Could you check a few things on this model? Use its own coordinates, in mm. Face numbers are marked on the shaded views. A direction names the side the tool comes from. Give positions to 0.01 mm unless a question says otherwise; leave off trailing zeros. Loops run counter-clockwise (first coordinate to the right, second up) from the corner with the lowest first, then second, coordinate; pieces in that order, holes last. Notation, with made-up numbers: M -8,8.5 L 14,8.5 A21 cw 14,44.5 Z; hole C 31.5,7.5 d7. An arc over 180 degrees is marked long. Answer in a Markdown table with one row per item. Add a question column.
1. If we section it at B-B on x = -8: List the corners of the cut face in (y, z) for me.
2. I'm going to push flat-ended pins straight in: pin 1 Ø1.8 at (x, z) = (-30, -45) entering from +Y; pin 2 Ø4.5 at (y, z) = (8, -41) entering from -X; pin 3 Ø7 at (x, z) = (-29, -39.5) entering from -Y; pin 4 Ø0.7 at (x, z) = (30, -45) entering from +Y. Where does each tip first touch, or does it pass through?
3. I need wall thicknesses on line 1 along X through (y, z) = (29.75, -45); line 2 along Z through (x, y) = (26, 15); line 3 along X through (y, z) = (24.5, 24.5). Which ranges of each line are inside material? Lowest first, please. Write a range as from..to.
4. Thinking about a two-plate mould opening in X: for the marked faces 5, 6, 7 and 8, which applies, released by +X, released by -X, zero draft, split by the parting line, or undercut?
5. Which directions (+Z, -Z, +X, -X, +Y, -Y) give clear straight access to the entire face, cutting with the end or side of a thin tool? Please do the marked faces 1, 2, 3 and 4.
6. If we section it at D-D on z = 19: List the corners of the cut face in (x, y) for me.
7. If we section it at A-A on y = 22: List the corners of the cut face in (x, z) for me, then the cut area to 3 significant figures.
8. If we section it at C-C on z = -42: List the corners of the cut face in (x, y) for me, then the cut area to 3 significant figures.
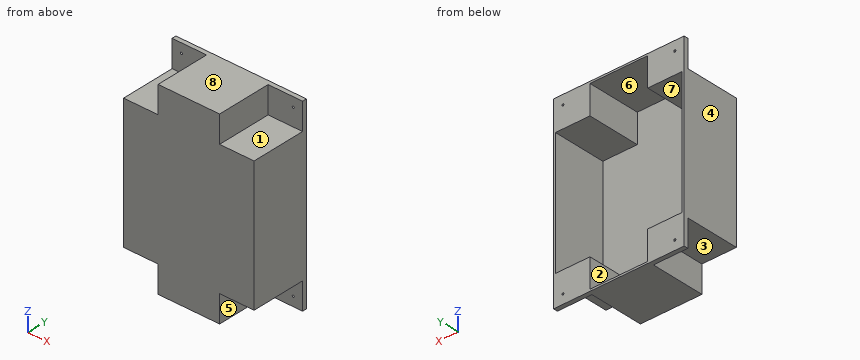
```python
from build123d import *

# Parameters (mm, degrees)
CROQUIS1_W              = 70
CROQUIS1_H              = 100
SALIENTE_EXTRUIR1_DEPTH = 3
CROQUIS2_W              = 70
CROQUIS2_H              = 100
SALIENTE_EXTRUIR2_DEPTH = 28.5
CROQUIS3_R              = 0.56
CORTAR_EXTRUIR1_DEPTH   = 69.682239334
CROQUIS4_W              = 18.5
CROQUIS4_H              = 14.45
CORTAR_EXTRUIR2_DEPTH   = 29.2


with BuildPart() as part:
    # Croquis1 → Saliente-Extruir1 (new body)
    with BuildSketch(Plane(origin=(0, 0, 0), x_dir=(1, 0, 0), z_dir=(0, 1, 0))):
        Rectangle(CROQUIS1_W, CROQUIS1_H)
    extrude(amount=SALIENTE_EXTRUIR1_DEPTH)

    # Croquis2 → Saliente-Extruir2 (add)
    with BuildSketch(Plane(origin=(0, 3, 0), x_dir=(1, 0, 0), z_dir=(0, 1, 0))):
        Rectangle(CROQUIS2_W, CROQUIS2_H)
        Polygon((-34, 33.55), (-15.5, 33.55), (-15.5, 49), (15.5, 49), (15.5, 33.55), (34, 33.55), (34, -33.55), (15.5, -33.55), (15.5, -49), (-15.5, -49), (-15.5, -33.55), (-34, -33.55), align=None, mode=Mode.SUBTRACT)
    extrude(amount=SALIENTE_EXTRUIR2_DEPTH)

    # Croquis3 → Cortar-Extruir1 (cut, through all)
    with BuildSketch(Plane.XZ):
        with Locations(Location((-30, -45, 0), (0, 0, 270))):
            Circle(CROQUIS3_R)
        with Locations(Location((-30, 45, 0), (0, 0, 90))):
            Circle(CROQUIS3_R)
        with Locations(Location((30, -45, 0), (0, 0, 90))):
            Circle(CROQUIS3_R)
        with Locations(Location((30, 45, 0), (0, 0, 270))):
            Circle(CROQUIS3_R)
    extrude(amount=-CORTAR_EXTRUIR1_DEPTH, mode=Mode.SUBTRACT)

    # Croquis4 → Cortar-Extruir2 (cut)
    with BuildSketch(Plane.XZ):
        with Locations((-25.75, 42.775)):
            Rectangle(CROQUIS4_W, CROQUIS4_H)
        with Locations((25.75, 42.775)):
            Rectangle(CROQUIS4_W, CROQUIS4_H)
        with Locations((25.75, -42.775)):
            Rectangle(CROQUIS4_W, CROQUIS4_H)
        with Locations((-25.75, -42.775)):
            Rectangle(CROQUIS4_W, CROQUIS4_H)
    extrude(amount=-CORTAR_EXTRUIR2_DEPTH, mode=Mode.SUBTRACT)


solid = part.part
```
Results:
| question | item | result |
|---|---|---|
| 1 | outline | M 0,-50 L 31.5,-50 L 31.5,-49 L 3,-49 L 3,49 L 31.5,49 L 31.5,50 L 0,50 Z |
| 2 | pin 1 | y = 31.5 |
| 2 | pin 2 | x = -16.5 |
| 2 | pin 3 | y = 29.2 |
| 2 | pin 4 | through |
| 3 | line 1 | -35..-30.56, -29.44..-15.5, 15.5..29.44, 30.56..35 |
| 3 | line 2 | -35.55..-33.55, 33.55..35.55 |
| 3 | line 3 | -35..-34, 34..35 |
| 4 | face 5 | released by +X |
| 4 | face 6 | undercut |
| 4 | face 7 | undercut |
| 4 | face 8 | zero draft |
| 5 | face 1 | +Z, +X, -Y |
| 5 | face 2 | +Y |
| 5 | face 3 | -Z, -X, -Y |
| 5 | face 4 | +Z, -Z, -X, +Y, -Y |
| 6 | outline | M -35,0 L 35,0 L 35,31.5 L 34,31.5 L 34,3 L -34,3 L -34,31.5 L -35,31.5 Z |
| 7 | outline | M -35,-35.55 L -16.5,-35.55 L -16.5,-50 L 16.5,-50 L 16.5,-35.55 L 35,-35.55 L 35,35.55 L 16.5,35.55 L 16.5,50 L -16.5,50 L -16.5,35.55 L -35,35.55 Z; hole M -34,-33.55 L -15.5,-33.55 L -15.5,-49 L 15.5,-49 L 15.5,-33.55 L 34,-33.55 L 34,33.55 L 15.5,33.55 L 15.5,49 L -15.5,49 L -15.5,33.55 L -34,33.55 Z |
| 7 | area | 410 mm2 |
| 8 | outline | M -35,29.2 L -16.5,29.2 L -16.5,0 L 16.5,0 L 16.5,29.2 L 35,29.2 L 35,31.5 L 15.5,31.5 L 15.5,3 L -15.5,3 L -15.5,31.5 L -35,31.5 Z |
| 8 | area | 241 mm2 |
